```python
from build123d import *

# Parameters (mm, degrees)
SALIENTE_EXTRUIR1_DEPTH = 8
REDONDEO1_R             = 4
CROQUIS6_R              = 2.8
CORTAR_EXTRUIR1_DEPTH   = 80.000001
CROQUIS7_R              = 1.5
CORTAR_EXTRUIR2_DEPTH   = 8
CORTAR_EXTRUIR3_DEPTH   = 3


with BuildPart() as part:
    # Croquis1 → Saliente-Extruir1 (new body)
    with BuildSketch(Plane.XY):
        Polygon((-96.284761278, 9.613034623), (-96.284761278, -70.386965377), (-104.284761278, -70.386965377), (-104.284761278, 49.613034623), (-96.284761278, 49.613034623), (-96.284761278, 19.613034623), (-32.284761278, 19.613034623), (-32.284761278, 49.613034623), (-24.284761278, 49.613034623), (-24.284761278, -70.386965377), (-32.284761278, -70.386965377), (-32.284761278, 9.613034623), align=None)
    extrude(amount=SALIENTE_EXTRUIR1_DEPTH)

    # Redondeo1
    redondeo1_edges = [part.edges().sort_by_distance(p)[0] for p in [
        (-100.284761278, -70.386965377, 0),
        (-28.284761278, -70.386965377, 0),
        (-28.284761278, 49.613034623, 8),
        (-28.284761278, 49.613034623, 0),
        (-100.284761278, 49.613034623, 0),
        (-100.284761278, 49.613034623, 8),
        (-28.284761278, -70.386965377, 8),
        (-100.284761278, -70.386965377, 8),
    ]]
    fillet(redondeo1_edges, radius=REDONDEO1_R - 0.0001)  # a hair under: the kernel refuses the full size

    # Croquis4 → Revolución3 (revolve)
    with BuildSketch(Plane.XY.offset(4), mode=Mode.PRIVATE) as revoluci_n3_sk:
        with BuildLine():
            Line((-104.284761278, 49.613034623), (-112.284761278, 49.613034623))
            ThreePointArc((-112.284761278, 49.613034623), (-115.113188403, 48.441461748), (-116.284761278, 45.613034623))
            Line((-116.284761278, 45.613034623), (-104.284761278, 45.613034623))
            Line((-104.284761278, 45.613034623), (-104.284761278, 49.613034623))
        make_face()
    revoluci_n3 = revolve(revoluci_n3_sk.sketch.rotate(Axis((-104.284761278, 45.613034623, 4), (-1, 0, 0)), 90), axis=Axis((-104.284761278, 45.613034623, 4), (-1, 0, 0)))

    # Simetría1: Revolución3 across plane
    add(revoluci_n3.mirror(Plane.ZY.offset(64.284761278)))

    # Croquis6 → Cortar-Extruir1 (cut)
    with BuildSketch(Plane.ZY.offset(104.284761278)):
        with Locations((8, 24.613034623)):
            Circle(CROQUIS6_R)
    extrude(amount=-CORTAR_EXTRUIR1_DEPTH, mode=Mode.SUBTRACT)

    # Croquis7 → Cortar-Extruir2 (cut)
    with BuildSketch(Plane.XY.offset(8)):
        with Locations((-100.284761278, 16.813034623)):
            Circle(CROQUIS7_R)
        with Locations((-28.284761278, 16.813034623)):
            Circle(CROQUIS7_R)
        with Locations((-28.284761278, 32.413034623)):
            Circle(CROQUIS7_R)
        with Locations((-100.284761278, 32.413034623)):
            Circle(CROQUIS7_R)
    extrude(amount=-CORTAR_EXTRUIR2_DEPTH, mode=Mode.SUBTRACT)

    # Croquis8 → Cortar-Extruir3 (cut)
    with BuildSketch(Plane(origin=(0, 0, 0), x_dir=(-1, 0, 0), z_dir=(0, 0, -1))):
        Polygon((103.748862893, 16.813034623), (102.016812085, 19.813034623), (98.55271047, 19.813034623), (96.820659663, 16.813034623), (98.55271047, 13.813034623), (102.016812085, 13.813034623), align=None)
        Polygon((31.748862893, 16.813034623), (30.016812085, 19.813034623), (26.55271047, 19.813034623), (24.820659663, 16.813034623), (26.55271047, 13.813034623), (30.016812085, 13.813034623), align=None)
        Polygon((103.748862893, 32.413034623), (102.016812085, 35.413034623), (98.55271047, 35.413034623), (96.820659663, 32.413034623), (98.55271047, 29.413034623), (102.016812085, 29.413034623), align=None)
        Polygon((31.748862893, 32.413034623), (30.016812085, 35.413034623), (26.55271047, 35.413034623), (24.820659663, 32.413034623), (26.55271047, 29.413034623), (30.016812085, 29.413034623), align=None)
    extrude(amount=-CORTAR_EXTRUIR3_DEPTH, mode=Mode.SUBTRACT)


solid = part.part
```
Part model, mm, in its own coordinate system. A direction names the side the tool comes from. Round coordinates to 2 decimals unless told otherwise and drop trailing zeros. Order: outer loops, then holes, each group sorted by start corner. A loop starts at its lowest first (then second) coordinate and runs counter-clockwise, first axis right, second up. Notation, with made-up numbers: M 49,53.5 L 66,53.5 A14 ccw 66,66.5 Z; hole C 18,74 d3. An arc over 180 degrees is marked long. Put each result on its own line as item: value. Start each with the question number.
1. Slice it at C-C on y = 26. List the corners of the cut face in (x, z), then the cut area to 3 significant figures.
2. Drill centre lines: probe 1 along X at (y, z) = (-40.5, 7.75); probe 2 along Y at (x, z) = (-57.5, 2.25); probe 3 along Y at (x, z) = (-24, 4.5). Where is each one in solid material? Low to high. Write a range as [from, to].
3. Slice it at D-D on z = 1.25. State how many separate pieces and enclosed holes the cut face has, then the cut area to 3 significant figures.
4. Tool access for faces 1 (the face through (-102.87, 15.29, 1.48)), 2 (the face through (-100.3, 24.7, 5.2)): list every direction of +Z, -Z, +X, -X, +Y, -Y with a clear straight run to the whole face (end or side of a thin tool).
5. Two-plate mould, pull along Y, no slides. Class faces 3 (the face through (-30.87, 30.89, 1.48)), 4 (the face through (-97.699, 33.934, 1.479)), 5 (the face through (-65, 19.613, 4)), 6 (the face through (-64, 9.613, 4)): +Y half, -Y half, draft (parallel to the pull), parting line (faces both ways), or undercut.
6. Slice it at B-B on x = -54. List the corners of the cut face in (y, z), then the cut area to 3 significant figures.
7. Drop flat-ended pins along their axis: pin 1 (1.5 mm diameter, centred on x = -27.5, z = 1.5, fed in from +Y); pin 2 (2.5 mm diameter, centred on x = -27.5, z = 1.5, fed in from -Y); pin 3 (4 mm diameter, centred on x = -100.28, y = 32.41, fed in from +Z); pin 4 (3 mm diameter, centred on y = 26.5, z = 5, fed in from -X). Give the stop position or say it passes through.
8. Slice it at A-A on y = 38.5. List the corners of the cut face in (x, z), then the cut area to 3 significant figures.
Findings:
1. outline: M -104.28,0 L -96.28,0 L -96.28,5.57 L -104.28,5.57 Z; M -32.28,0 L -24.28,0 L -24.28,5.57 L -32.28,5.57 Z
1. area: 89.1 mm2
2. probe 1: [-104.28, -96.28], [-32.28, -24.28]
2. probe 2: [9.61, 19.61]
2. probe 3: [41.64, 49.58]
3. separate pieces: 1
3. enclosed holes: 4
3. area: 2,520 mm2
4. face 1: -Z
4. face 2: +Z, +X, -X
5. face 3: undercut
5. face 4: undercut
5. face 5: +Y half
5. face 6: -Y half
6. outline: M 9.61,0 L 19.61,0 L 19.61,8 L 9.61,8 Z
6. area: 80.0 mm2
7. pin 1: y = 49.21
7. pin 2: y = -70.19
7. pin 3: z = 8
7. pin 4: x = -104.28
8. outline: M -104.28,0 L -96.28,0 L -96.28,8 L -104.28,8 Z; M -32.28,0 L -24.28,0 L -24.28,8 L -32.28,8 Z
8. area: 128 mm2
